from build123d import *

# Parameters (mm, degrees)
F0_R     = 158.5
F0_R_2   = 145
F1_DEPTH = 125
F2_R     = 158.5
F3_DEPTH = 30
F4_SIZE  = 25
F5_DEPTH = 20


with BuildPart() as f1:
    # F0 (on Front) → F1 (new body)
    with BuildSketch(Plane.XZ):
        Circle(F0_R)
        Circle(F0_R_2, mode=Mode.SUBTRACT)
    extrude(amount=F1_DEPTH)

    # F2 (on face) → F3 (join)
    with BuildSketch(Plane(origin=(0, 0, 0), x_dir=(-1, 0, 0), z_dir=(0, 1, 0))):
        Circle(F2_R)
    extrude(amount=-F3_DEPTH)

    # F4
    f4_edges = [f1.edges().sort_by_distance(p)[0] for p in [
        (-158.5, 0, 0),
    ]]
    chamfer(f4_edges, length=F4_SIZE)

    # F5 (add): a face of the model
    f5_faces = [f1.faces().sort_by_distance(p)[0] for p in [
        (-154.0169430073, -125, 0),
    ]]
    extrude(f5_faces, amount=F5_DEPTH)


solid = f1.part
Model file for the job. Use its own axes, mm. A direction names the side the tool comes from. Give positions to 0.01 mm unless a question says otherwise; leave off trailing zeros. Order: outer loops, then holes, each group sorted by start corner. A loop starts at its lowest first (then second) coordinate and runs counter-clockwise, first axis right, second up. Notation, with made-up numbers: M 40,66 L 54,66 A20 cw 54,87 Z; hole C -12,68.5 d3. An arc over 180 degrees is marked long. Put each result on its own line as item: value. Start each with the question number.
(1) Band-saw the part on C-C on y = -99.5. Give the cut face in (x, z), then the cut area to 3 significant figures.
(2) Band-saw the part on B-B on z = 0. Give the cut face in (x, y), then the cut area to 3 significant figures.
(3) Band-saw the part on D-D on y = -14.5. Give the cut face in (x, z), then the cut area to 3 significant figures.
(4) Pull direction Z, two halves, no side cores. Call faces 1 (the face through (-29.2, -1.21, -131.51)), 2 (the face through (-2, 0, 2)), 3 (the face through (138.304, -86.695, 43.554)): released by +Z, released by -Z, zero draft, split by the parting line, or undercut.
(5) Drill centre lines: L1, parallel to Z at x = 0, y = -113.5; L2, parallel to X at y = -93.5, z = -4.5; L3, parallel to Y at x = 89, z = -73. Where is each one in solid material? Low to high. Write a range as [from, to].
(6) Band-saw the part on A-A on x = 0. Give the cut face in (y, z).
(7) Tool access for faces 4 (the face through (128, -145, -70)), 5 (the face through (2, -30, 2)): list every direction of +Z, -Z, +X, -X, +Y, -Y with a clear straight run to the whole face (end or side of a thin tool).
(8) Pin check, flat tips, straight feed: pin 1 Ø1.5 at (x, y) = (73, -41.5) entering from -Z; pin 2 Ø10 at (x, y) = (-82.5, -128.5) entering from +Z; pin 3 Ø8 at (x, y) = (-25.5, -46.5) entering from -Z (3 decimals). Stop position of each tip, or through.
Results below:
1. outline: C 0,0 d317; hole C 0,0 d290
1. area: 12,900 mm2
2. outline: M -158.5,-145 L -145,-145 L -145,-30 L 145,-30 L 145,-145 L 158.5,-145 L 158.5,-25 L 133.5,0 L -133.5,0 L -158.5,-25 Z
2. area: 12,000 mm2
3. outline: C 0,0 d296
3. area: 68,800 mm2
4. face 1: split by the parting line
4. face 2: zero draft
4. face 3: undercut
5. L1: z = [-158.5, -145], [145, 158.5]
5. L2: x = [-158.44, -144.93], [144.93, 158.44]
5. L3: y = [-30, 0]
6. outline: M -145,-158.5 L -25,-158.5 L 0,-133.5 L 0,133.5 L -25,158.5 L -145,158.5 L -145,145 L -30,145 L -30,-145 L -145,-145 Z
7. face 4: +Z, -Z, +X, -X, -Y
7. face 5: -Y
8. pin 1: stops at z = -141.08
8. pin 2: stops at z = 138.26
8. pin 3: stops at z = -157.035
